Study the drawing (mm; zero at the part's minimum x, y, z) and answer. A direction names the side the tool comes from. Coordinates: 2 decimals unless noted, no trailing zeros. Order: outer loops, then holes, each group sorted by start corner. A loop starts at its lowest first (then second) coordinate and runs counter-clockwise, first axis right, second up. Notation, with made-up numbers: (41.5, 22.5) -> (45.5, 22.5) arc R9 ccw to (45.5, 32.5) -> close; hole circle Ø2 at (-10, 49). An arc over 180 degrees is marked (long way). Answer as CSV lines item,"result". Start each with the question number.
Item 1: Section C-C (y = 20.5) is taken. Write down the section's boundary in (x, z), then the cut area to 3 significant figures.
Item 2: Each of these flat-tipped pins is pushed along its axis until it touches: pin 1 Ø6 at (y, z) = (6.5, 23) entering from +X; pin 2 Ø8 at (y, z) = (11.5, 26.5) entering from -X; pin 3 Ø1.2 at (y, z) = (1.5, 70.5) entering from -X; pin 4 Ø12 at (y, z) = (20, 53) entering from -X. Where does it stop, or does it pass through?
Item 3: Straight lines are drawn through the part: L1, parallel to X at y = 15.25, z = 55; L2, parallel to Z at x = 23, y = 3.75. For each, find the intervals that lie inside material, in ascending order.
Item 4: Section A-A (z = 62.5) is taken. Write down the section's boundary in (x, y), then the cut area to 3 significant figures.
Item 5: Section B-B (x = 31) is taken. Write down the section's boundary in (y, z), then the cut area to 3 significant figures.
Item 6: Section D-D (z = 17) is taken. Write down the section's boundary in (x, y).
Item 7: Which of the six approach directions +Z, -Z, +X, -X, +Y, -Y give full straight-line access (tool end or side, diameter ignored) to the marked faces 1 and 2?
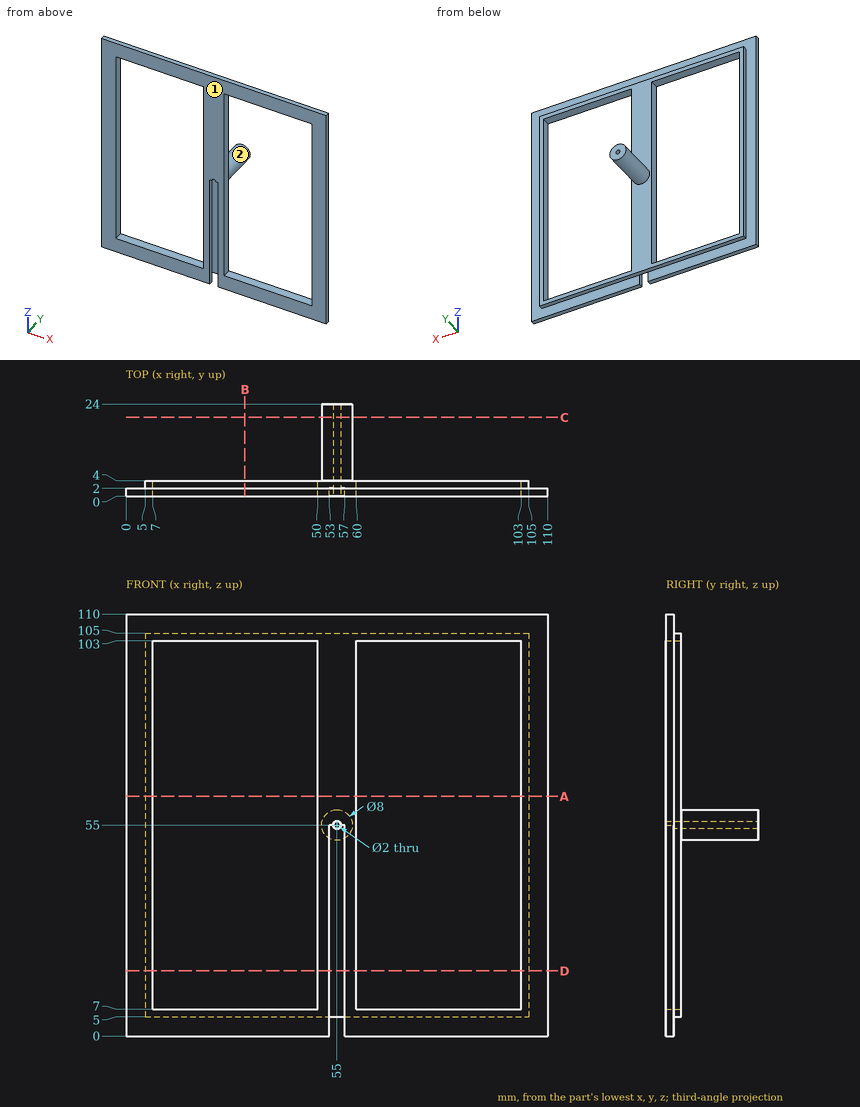
Checked values:
1,outline,"circle Ø8 at (55, 55); hole circle Ø2 at (55, 55)"
1,area,"47.1 mm^2"
2,pin 1,"stops at x = 105"
2,pin 2,"passes through"
2,pin 3,"stops at x = 0"
2,pin 4,"stops at x = 51"
3,L1,"x = 51 to 54, 56 to 59"
3,L2,"z = 5 to 7, 103 to 105"
4,outline,"(0, 0) -> (7, 0) -> (7, 4) -> (5, 4) -> (5, 2) -> (0, 2) -> close; (50, 0) -> (60, 0) -> (60, 4) -> (50, 4) -> close; (103, 0) -> (110, 0) -> (110, 2) -> (105, 2) -> (105, 4) -> (103, 4) -> close"
4,area,"76.0 mm^2"
5,outline,"(0, 0) -> (2, 0) -> (2, 5) -> (4, 5) -> (4, 7) -> (0, 7) -> close; (0, 103) -> (4, 103) -> (4, 105) -> (2, 105) -> (2, 110) -> (0, 110) -> close"
5,area,"36.0 mm^2"
6,outline,"(0, 0) -> (7, 0) -> (7, 4) -> (5, 4) -> (5, 2) -> (0, 2) -> close; (50, 0) -> (53, 0) -> (53, 2) -> (57, 2) -> (57, 0) -> (60, 0) -> (60, 4) -> (50, 4) -> close; (103, 0) -> (110, 0) -> (110, 2) -> (105, 2) -> (105, 4) -> (103, 4) -> close"
7,face 1,"+Z, -Z, +X, -X, -Y"
7,face 2,"+Y"
